```python
from build123d import *

# Parameters (mm, degrees)
BOSS_EXTRUDE1_DEPTH      = 75
SKETCH2_R                = 1.1
CUT_EXTRUDE1_DEPTH       = 121.933866224
BOSS_EXTRUDE2_DEPTH      = 2.458497378
SKETCH4_R                = 1.1
CUT_EXTRUDE2_DEPTH       = 121.933866224
SKETCH5_W                = 20
SKETCH5_H                = 2.5
CUT_EXTRUDE3_DEPTH       = 2
CUT_EXTRUDE4_DEPTH       = 121.933866224
CUT_EXTRUDE4_DEPTH_BACK  = 2.55
SKETCH6_W                = 17.78
SKETCH6_H                = 2.54
SKETCH7_W                = 1
SKETCH7_H                = 0.979795898
CUT_EXTRUDE5_DEPTH       = 121.113488002
SKETCH8_W                = 0.635
SKETCH8_H                = 0.635
CUT_EXTRUDE6_DEPTH       = 121.113488002
BOSS_EXTRUDE3_DEPTH      = 2
BOSS_EXTRUDE3_DEPTH_BACK = 1
SKETCH9_W                = 24
SKETCH9_H                = 25
FILLET1_R                = 2
SKETCH10_R               = 1
CUT_EXTRUDE7_DEPTH       = 4
SKETCH11_W               = 8
SKETCH11_H               = 4
CUT_EXTRUDE8_DEPTH       = 1
FILLET2_R                = 2
SKETCH12_R               = 1.25
SKETCH12_R_2             = 1.47
CUT_EXTRUDE10_DEPTH      = 3.5


with BuildPart() as part:
    # Sketch1 → Boss-Extrude1 (new body)
    with BuildSketch(Plane(origin=(0, 0, 0), x_dir=(1, 0, 0), z_dir=(0, 1, 0))):
        Polygon((23.5, 30), (23.5, 26.5), (3.5, 26.5), (3.5, 3.5), (86.5, 3.5), (86.5, 26.5), (66.5, 26.5), (66.5, 30), (90, 30), (90, 0), (0, 0), (0, 30), align=None)
    extrude(amount=BOSS_EXTRUDE1_DEPTH)

    # Sketch2 → Cut-Extrude1 (cut, through all)
    with BuildSketch(Plane.XY):
        with Locations((53, 10)):
            Circle(SKETCH2_R)
        with Locations((37, 10)):
            Circle(SKETCH2_R)
    extrude(amount=-CUT_EXTRUDE1_DEPTH, mode=Mode.SUBTRACT)

    # Sketch3 → Boss-Extrude2 (add)
    with BuildSketch(Plane.XY):
        with BuildLine():
            Line((53, 13), (37, 13))
            ThreePointArc((37, 13), (34, 10), (37, 7))
            Line((37, 7), (53, 7))
            ThreePointArc((53, 7), (56, 10), (53, 13))
        make_face()
    extrude(amount=BOSS_EXTRUDE2_DEPTH)

    # Sketch4 → Cut-Extrude2 (cut, through all)
    with BuildSketch(Plane(origin=(0, 0, 0), x_dir=(-1, 0, 0), z_dir=(0, 0, -1))):
        with Locations(Location((-37, 10, 0), (0, 0, 180))):
            Circle(SKETCH4_R)
        with Locations(Location((-53, 10, 0), (0, 0, 180))):
            Circle(SKETCH4_R)
    extrude(amount=-CUT_EXTRUDE2_DEPTH, mode=Mode.SUBTRACT)

    # Sketch5 → Cut-Extrude3 (cut)
    with BuildSketch(Plane.XY):
        with Locations((44.985, 26.3)):
            Rectangle(SKETCH5_W, SKETCH5_H)
    extrude(amount=-CUT_EXTRUDE3_DEPTH, mode=Mode.SUBTRACT)

    # Sketch6 → Cut-Extrude4 (cut, two sides: drawn at the far end of the back side and taken through both)
    with BuildSketch(Plane.XY.offset(-CUT_EXTRUDE4_DEPTH_BACK)):
        with Locations((44.99, 51.27)):
            Rectangle(SKETCH6_W, SKETCH6_H)
    extrude(amount=CUT_EXTRUDE4_DEPTH + CUT_EXTRUDE4_DEPTH_BACK, mode=Mode.SUBTRACT)

    # Sketch7 → Cut-Extrude5 (cut, through all)
    with BuildSketch(Plane(origin=(0, 0, -3.5), x_dir=(-1, 0, 0), z_dir=(0, 0, -1))):
        with Locations((-53.765, 26.2)):
            Rectangle(SKETCH7_W, SKETCH7_H)
        with Locations((-51.245, 26.2)):
            Rectangle(SKETCH7_W, SKETCH7_H)
        with Locations((-48.735, 26.2)):
            Rectangle(SKETCH7_W, SKETCH7_H)
        with Locations((-46.215, 26.2)):
            Rectangle(SKETCH7_W, SKETCH7_H)
        with Locations((-43.705, 26.2)):
            Rectangle(SKETCH7_W, SKETCH7_H)
        with Locations((-41.195, 26.2)):
            Rectangle(SKETCH7_W, SKETCH7_H)
        with Locations((-38.685, 26.2)):
            Rectangle(SKETCH7_W, SKETCH7_H)
        with Locations((-36.175, 26.2)):
            Rectangle(SKETCH7_W, SKETCH7_H)
    extrude(amount=-CUT_EXTRUDE5_DEPTH, mode=Mode.SUBTRACT)

    # Sketch8 → Cut-Extrude6 (cut, through all)
    with BuildSketch(Plane(origin=(0, 0, -3.5), x_dir=(-1, 0, 0), z_dir=(0, 0, -1))):
        with Locations((-52.61, 51.27)):
            Rectangle(SKETCH8_W, SKETCH8_H)
        with Locations((-50.07, 51.27)):
            Rectangle(SKETCH8_W, SKETCH8_H)
        with Locations((-47.53, 51.27)):
            Rectangle(SKETCH8_W, SKETCH8_H)
        with Locations((-44.99, 51.27)):
            Rectangle(SKETCH8_W, SKETCH8_H)
        with Locations((-42.45, 51.27)):
            Rectangle(SKETCH8_W, SKETCH8_H)
        with Locations((-39.91, 51.27)):
            Rectangle(SKETCH8_W, SKETCH8_H)
        with Locations((-37.37, 51.27)):
            Rectangle(SKETCH8_W, SKETCH8_H)
    extrude(amount=-CUT_EXTRUDE6_DEPTH, mode=Mode.SUBTRACT)

    # Sketch9 → Boss-Extrude3 (add, two sides: drawn at the far end of the back side and taken through both)
    with BuildSketch(Plane.XZ.offset(-BOSS_EXTRUDE3_DEPTH_BACK)):
        with Locations((45, -8.5)):
            Rectangle(SKETCH9_W, SKETCH9_H)
    extrude(amount=BOSS_EXTRUDE3_DEPTH + BOSS_EXTRUDE3_DEPTH_BACK)

    # Fillet1
    fillet1_edges = [part.edges().sort_by_distance(p)[0] for p in [
        (57, -0.5, 4),
        (33, -0.5, -21),
        (57, -0.5, -21),
        (33, -0.5, 4),
    ]]
    fillet(fillet1_edges, radius=FILLET1_R)

    # Sketch10 → Cut-Extrude7 (cut)
    with BuildSketch(Plane.XZ.offset(2)):
        with Locations((47.5, -19)):
            Circle(SKETCH10_R)
        with Locations((35, -19)):
            Circle(SKETCH10_R)
        with Locations((47.5, 2)):
            Circle(SKETCH10_R)
        with Locations((35, 2)):
            Circle(SKETCH10_R)
    extrude(amount=-CUT_EXTRUDE7_DEPTH, mode=Mode.SUBTRACT)

    # Sketch11 → Cut-Extrude8 (cut)
    with BuildSketch(Plane(origin=(0, 1, 0), x_dir=(1, 0, 0), z_dir=(0, 1, 0))):
        with Locations((47.5, -2)):
            Rectangle(SKETCH11_W, SKETCH11_H)
    extrude(amount=-CUT_EXTRUDE8_DEPTH, mode=Mode.SUBTRACT)

    # Fillet2
    fillet2_edges = [part.edges().sort_by_distance(p)[0] for p in [
        (0, 37.5, -30),
        (3.5, 37.5, -26.5),
        (3.5, 37.5, -3.5),
        (86.5, 37.5, -3.5),
        (86.5, 37.5, -26.5),
        (90, 37.5, -30),
        (90, 37.5, 0),
        (0, 37.5, 0),
    ]]
    fillet(fillet2_edges, radius=FILLET2_R)

    # Sketch12 → Cut-Extrude10 (cut)
    with BuildSketch(Plane.XY):
        with Locations((79.735, 27.5)):
            Circle(SKETCH12_R)
        with Locations((65.765, 27.5)):
            Circle(SKETCH12_R)
        with Locations((60.735, 27.5)):
            Circle(SKETCH12_R)
        with Locations((10.235, 27.5)):
            Circle(SKETCH12_R)
        with Locations((52.864, 67.714)):
            Circle(SKETCH12_R_2)
        with Locations((37.136, 67.714)):
            Circle(SKETCH12_R_2)
    extrude(amount=-CUT_EXTRUDE10_DEPTH, mode=Mode.SUBTRACT)


solid = part.part
```
Here's how the part is built. I have some questions about the finished solid (model axes, mm). A direction names the side the tool comes from. Round coordinates to 2 decimals unless told otherwise and drop trailing zeros. Loops run counter-clockwise (first coordinate to the right, second up) from the corner with the lowest first, then second, coordinate; pieces in that order, holes last. Notation, with made-up numbers: (12.25, -12.5) -> (61.25, -12.5) arc R29 cw to (61.25, 26.5) -> close; hole circle Ø4 at (72.25, 47.5). An arc over 180 degrees is marked (long way). Answer as CSV lines item,"result". Start each with the question number.
1. I'm going to push flat-ended pins straight in: P1, Ø6, axis at x = 73.5, y = 66.5, coming from the +Z side; P2, Ø1.1, axis at y = 0.5, z = 1, coming from the -X side; P3, Ø1, axis at x = 39.5, y = 53.5, coming from the -Z side; P4, Ø9, axis at x = 73, z = -18.5, coming from the -Y side. Where does each tip first touch, or does it pass through?
2. Imagine slicing it at B-B on x = 15.5. Write out the boundary of the cut face in (y, z), plus the area to 3 significant figures.
3. I need wall thicknesses on probe 1 along X at (y, z) = (58, -6); probe 2 along Z at (x, y) = (77, 67); probe 3 along X at (y, z) = (10, -1). Which ranges of each line are inside material? Lowest first, please. Write a range as from..to.
4. Imagine slicing it at D-D on x = 30. Write out the boundary of the cut face in (y, z), plus the area to 4 significant figures.
5. Imagine slicing it at A-A on z = -13. Write out the boundary of the cut face in (x, y), plus the area to 3 significant figures.
6. For faces 1 (the face through (54.985, 26, -1)), 2 (the face through (56, 10, 1)), 3 (the face through (4.07, 38.02, -25.9)), 4 (the face through (89.43, 38.02, -29.4)), 5 (the face through (33.57, -0.52, -20.4)), which set-ups out of +Z, -Z, +X, -X, +Y, -Y let a thin tool reach every point of the face, with its end or its side?
7. If we mould it in two halves opening along Y, with no side actions, what happens to faces 6 (the face through (34, 10, 1)), 7 (the face through (48.454, -1.014, 2.3)), 8 (the face through (3, 0, -13))? For each: pulls with the +Y half, pulls with the -Y half, needs draft (parallel to the pull), parting line crosses it, or undercut.
8. Imagine slicing it at C-C on y = 49. Write out the boundary of the cut face in (x, z), plus the area to 4 significant figures.
Solution:
1,P1,"z = 0"
1,P2,"x = 33"
1,P3,"z = -3.5"
1,P4,"through"
2,outline,"(0, -30) -> (75, -30) -> (75, -26.5) -> (0, -26.5) -> close; (0, -3.5) -> (75, -3.5) -> (75, 0) -> (0, 0) -> close"
2,area,"525 mm²"
3,probe 1,"0..3.5, 86.5..90"
3,probe 2,"-30..-26.5, -3.5..0"
3,probe 3,"0.27..35.9, 38.1..51.9, 54.1..89.73"
4,outline,"(0, -3.5) -> (75, -3.5) -> (75, 0) -> (0, 0) -> close"
4,area,"262.5 mm²"
5,outline,"(0, 0) -> (3.5, 0) -> (3.5, 75) -> (0, 75) -> close; (33, -2) -> (57, -2) -> (57, 1) -> (33, 1) -> close; (86.5, 0) -> (90, 0) -> (90, 75) -> (86.5, 75) -> close"
5,area,"597 mm²"
6,face 1,"+Z"
6,face 2,"+Z, +X"
6,face 3,"+Y, -Y"
6,face 4,"-Z, +X, +Y, -Y"
6,face 5,"-Z, +Y, -Y"
7,face 6,"undercut"
7,face 7,"needs draft"
7,face 8,"pulls with the -Y half"
8,outline,"(0, -28) arc R2 ccw to (2, -30) -> (23.5, -30) -> (23.5, -26.5) -> (5.5, -26.5) arc R2 cw to (3.5, -24.5) -> (3.5, -5.5) arc R2 cw to (5.5, -3.5) -> (84.5, -3.5) arc R2 cw to (86.5, -5.5) -> (86.5, -24.5) arc R2 cw to (84.5, -26.5) -> (66.5, -26.5) -> (66.5, -30) -> (88, -30) arc R2 ccw to (90, -28) -> (90, -2) arc R2 ccw to (88, 0) -> (2, 0) arc R2 ccw to (0, -2) -> close"
8,area,"640.5 mm²"
